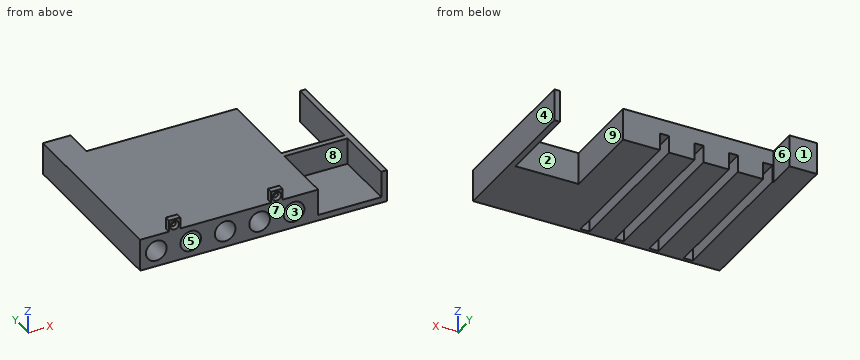
```python
from build123d import *

# Parameters (mm, degrees)
CYLINDER004_R     = 9
CYLINDER004_DEPTH = 130
CYLINDER003_R     = 9
CYLINDER003_DEPTH = 130
CYLINDER002_R     = 9
CYLINDER002_DEPTH = 130
CYLINDER001_R     = 9
CYLINDER001_DEPTH = 130
CYLINDER_R        = 9
CYLINDER_DEPTH    = 156
BOX007_W          = 8
BOX007_H          = 165
BOX007_DEPTH      = 15
BOX006_W          = 8
BOX006_H          = 165
BOX006_DEPTH      = 15
BOX005_W          = 8
BOX005_H          = 165
BOX005_DEPTH      = 15
BOX004_W          = 8
BOX004_H          = 165
BOX004_DEPTH      = 15
BOX003_W          = 197
BOX003_H          = 103
BOX003_DEPTH      = 33
BOX002_W          = 55
BOX002_H          = 103
BOX002_DEPTH      = 34
BOX001_W          = 55
BOX001_H          = 55
BOX001_DEPTH      = 23
BOX_W             = 215
BOX_H             = 159
BOX_DEPTH         = 28
PAD_DEPTH         = 5
HOLE_D            = 3.9
HOLE_DEPTH        = 25
HOLE_CSINK_D      = 7.8
HOLE_CSINK_ANGLE  = 90


with BuildPart() as cylinder004:
    # Cylinder004 → Cylinder004 (new body)
    with BuildSketch(Plane(origin=(134, 130, 14), x_dir=(1, 0, 0), z_dir=(0, -1, 0))):
        Circle(CYLINDER004_R)
    extrude(amount=CYLINDER004_DEPTH)


with BuildPart() as cylinder003:
    # Cylinder003 → Cylinder003 (new body)
    with BuildSketch(Plane(origin=(104, 130, 14), x_dir=(1, 0, 0), z_dir=(0, -1, 0))):
        Circle(CYLINDER003_R)
    extrude(amount=CYLINDER003_DEPTH)


with BuildPart() as cylinder002:
    # Cylinder002 → Cylinder002 (new body)
    with BuildSketch(Plane(origin=(74, 130, 14), x_dir=(1, 0, 0), z_dir=(0, -1, 0))):
        Circle(CYLINDER002_R)
    extrude(amount=CYLINDER002_DEPTH)


with BuildPart() as cylinder001:
    # Cylinder001 → Cylinder001 (new body)
    with BuildSketch(Plane(origin=(44, 130, 14), x_dir=(1, 0, 0), z_dir=(0, -1, 0))):
        Circle(CYLINDER001_R)
    extrude(amount=CYLINDER001_DEPTH)


with BuildPart() as cylinder:
    # Cylinder → Cylinder (new body)
    with BuildSketch(Plane(origin=(14, 156, 14), x_dir=(1, 0, 0), z_dir=(0, -1, 0))):
        Circle(CYLINDER_R)
    extrude(amount=CYLINDER_DEPTH)


with BuildPart() as cube007:
    # Box007 → Box007 (new body)
    with BuildSketch(Plane(origin=(115, 3, 0), x_dir=(1, 0, 0), z_dir=(0, 0, 1))):
        with Locations((4, 82.5)):
            Rectangle(BOX007_W, BOX007_H)
    extrude(amount=BOX007_DEPTH)


with BuildPart() as cube006:
    # Box006 → Box006 (new body)
    with BuildSketch(Plane(origin=(85, 3, 0), x_dir=(1, 0, 0), z_dir=(0, 0, 1))):
        with Locations((4, 82.5)):
            Rectangle(BOX006_W, BOX006_H)
    extrude(amount=BOX006_DEPTH)


with BuildPart() as cube005:
    # Box005 → Box005 (new body)
    with BuildSketch(Plane(origin=(55, 3, 0), x_dir=(1, 0, 0), z_dir=(0, 0, 1))):
        with Locations((4, 82.5)):
            Rectangle(BOX005_W, BOX005_H)
    extrude(amount=BOX005_DEPTH)


with BuildPart() as cube004:
    # Box004 → Box004 (new body)
    with BuildSketch(Plane(origin=(25, 3, 0), x_dir=(1, 0, 0), z_dir=(0, 0, 1))):
        with Locations((4, 82.5)):
            Rectangle(BOX004_W, BOX004_H)
    extrude(amount=BOX004_DEPTH)


with BuildPart() as cube003:
    # Box003 → Box003 (new body)
    with BuildSketch(Plane(origin=(24, 133, -3), x_dir=(1, 0, 0), z_dir=(0, 0, 1))):
        with Locations((98.5, 51.5)):
            Rectangle(BOX003_W, BOX003_H)
    extrude(amount=BOX003_DEPTH)


with BuildPart() as cube002:
    # Box002 → Box002 (new body)
    with BuildSketch(Plane(origin=(155, 60, -3), x_dir=(1, 0, 0), z_dir=(0, 0, 1))):
        with Locations((27.5, 51.5)):
            Rectangle(BOX002_W, BOX002_H)
    extrude(amount=BOX002_DEPTH)


with BuildPart() as cube001:
    # Box001 → Box001 (new body)
    with BuildSketch(Plane(origin=(155, 0, 5), x_dir=(1, 0, 0), z_dir=(0, 0, 1))):
        with Locations((27.5, 27.5)):
            Rectangle(BOX001_W, BOX001_H)
    extrude(amount=BOX001_DEPTH)


with BuildPart() as cut011:
    # Box → Box (new body)
    with BuildSketch(Plane.XY):
        with Locations((107.5, 79.5)):
            Rectangle(BOX_W, BOX_H)
    extrude(amount=BOX_DEPTH)

    # Cut: cut Cube001
    add(cube001.part, mode=Mode.SUBTRACT)

    # Cut001: cut Cube002
    add(cube002.part, mode=Mode.SUBTRACT)

    # Cut002: cut Cube003
    add(cube003.part, mode=Mode.SUBTRACT)

    # Cut003: cut Cube004
    add(cube004.part, mode=Mode.SUBTRACT)

    # Cut004: cut Cube005
    add(cube005.part, mode=Mode.SUBTRACT)

    # Cut005: cut Cube006
    add(cube006.part, mode=Mode.SUBTRACT)

    # Cut006: cut Cube007
    add(cube007.part, mode=Mode.SUBTRACT)

    # Cut007: cut Cylinder
    add(cylinder.part, mode=Mode.SUBTRACT)

    # Cut008: cut Cylinder001
    add(cylinder001.part, mode=Mode.SUBTRACT)

    # Cut009: cut Cylinder002
    add(cylinder002.part, mode=Mode.SUBTRACT)

    # Cut010: cut Cylinder003
    add(cylinder003.part, mode=Mode.SUBTRACT)

    # Cut011: cut Cylinder004
    add(cylinder004.part, mode=Mode.SUBTRACT)


with BuildPart() as fusion:
    # Sketch → Pad (new body)
    with BuildSketch(Plane.XZ):
        Polygon((25, 38), (35, 38), (35, 28), (114, 28), (114, 38), (124, 38), (124, 27), (114, 27), (35, 27), (25, 27), align=None)
    extrude(amount=PAD_DEPTH)

    # Hole
    with Locations(Plane.XZ.offset(5)):
        with Locations((30, 32.5), (119, 32.5)):
            CounterSinkHole(HOLE_D / 2, HOLE_CSINK_D / 2, depth=HOLE_DEPTH, counter_sink_angle=HOLE_CSINK_ANGLE)


with BuildPart() as fusion_1:
    # Body placement: moved
    add(fusion.part.moved(Location((0, 5, 0))))

    # Fusion: union Cut011
    add(cut011.part)


solid = fusion_1.part
```
Check sheet for the modelled part. Datum: model origin and axes. Units: mm. Face numbers are marked on the shaded views. A direction names the side the tool comes from. Round coordinates to 2 decimals unless told otherwise and drop trailing zeros. Loops run counter-clockwise (first coordinate to the right, second up) from the corner with the lowest first, then second, coordinate; pieces in that order, holes last. Notation, with made-up numbers: (3.5, 79.5) - (47.5, 79.5) arc R25 cw to (47.5, 113.5) - close; hole circle Ø11 at (37, 30). An arc over 180 degrees is marked (long way). Answer as a JSON object with one key per item and string values. Group by question number.
Q1. Gauge pin test, flat ends, axial feed: P1, Ø5, axis at x = 119, z = 32.5, coming from the +Y side; P2, Ø4, axis at x = 119, y = 75, coming from the -Z side; P3, Ø2, axis at x = 160.5, y = 62, coming from the +Z side; P4, Ø5.5, axis at y = 1.5, z = 35, coming from the -X side. Record the tip position at first contact, or that the pin passes through.
Q2. Sectioned sample at D-D, the plane x = 197. Enter the section's corners in (y, z).
Q3. Sectioned sample at A-A, the plane y = 123.5. Count the separate pieces of the cut face and the enclosed holes in it, plus the area to 3 significant figures.
Q4. Set-up check for the marked faces 5, 6, 7, 8 and 9: record each of +Z, -Z, +X, -X, +Y, -Y from which the full face is reachable in a straight line by a thin tool's end or side.
Q5. Scan lines: line 1 along X through (y, z) = (132.5, 2); line 2 along Z through (x, y) = (134, 79); line 3 along Z through (x, y) = (30, 3.9). Record each from-to range of solid material in increasing order. Write a range as [from, to].
Q6. Sectioned sample at B-B, the plane x = 44. Enter the section's corners in (y, z), plus the area to 3 significant figures.
Q7. Mould release check, pull along X, two halves, no side actions. Record for the marked faces 1, 2, 3 and 4: released by +X, released by -X, zero draft, split by the parting line, or undercut.
Solution:
{
 "1": {"P1": "stops at y = 5", "P2": "stops at z = 15", "P3": "passes through", "P4": "stops at x = 25"},
 "2": {"outline": "(0, 0) - (60, 0) - (60, 28) - (55, 28) - (55, 5) - (0, 5) - close"},
 "3": {"separate pieces": "2", "enclosed holes": "5", "area": "2,730 mm²"},
 "4": {"face 5": "-Y", "face 6": "+Z, -Z, +X, +Y", "face 7": "+Z, -Z, +X, -X, -Y", "face 8": "+Z, -Y", "face 9": "+Z, -Z, +Y"},
 "5": {"line 1": "x = [0, 25], [33, 55], [63, 85], [93, 115], [123, 155], [210, 215]", "line 2": "z = [0, 5], [23, 28]", "line 3": "z = [15, 30.55], [34.45, 38]"},
 "6": {"outline": "(0, 0) - (133, 0) - (133, 28) - (0, 28) - (0, 23) - (130, 23) - (130, 5) - (0, 5) - close", "area": "1,380 mm²"},
 "7": {"face 1": "zero draft", "face 2": "undercut", "face 3": "undercut", "face 4": "released by +X"}
}
